Geometry: final body of the model. Coordinates: model frame, mm. A direction names the side the tool comes from. Give positions to 0.01 mm unless a question says otherwise; leave off trailing zeros. Loops run counter-clockwise (first coordinate to the right, second up) from the corner with the lowest first, then second, coordinate; pieces in that order, holes last. Notation, with made-up numbers: (73, 45) - (107, 45) arc R18 cw to (107, 73) - close; hole circle Ø11 at (74.5, 86.5). An arc over 180 degrees is marked (long way). Answer in a Markdown table with one row per item.
from build123d import *

# Parameters (mm, degrees)
F1_DEPTH = 5
F2_R     = 37.5
F3_DEPTH = 10
F4_DEPTH = 40.7
F6_DEPTH = 15


with BuildPart() as f1:
    # F0 (on Top) → F1 (new body)
    with BuildSketch(Plane.XY):
        with BuildLine():
            Line((10, -10), (41.306779, -10))
            ThreePointArc((41.306779, -10), (-39.719354, 15.120281), (37.5, -20))
            Line((37.5, -20), (0, -20))
            Line((0, -20), (0, -5))
            ThreePointArc((0, -5), (-5, 0), (0, 5))
            Line((0, 5), (0, 20))
            ThreePointArc((0, 20), (5, 25), (10, 20))
            Line((10, 20), (10, 5))
            ThreePointArc((10, 5), (15, 0), (10, -5))
            Line((10, -5), (10, -10))
        make_face()
        with BuildLine():
            ThreePointArc((37.5, -20), (39.719354, -15.120281), (41.306779, -10))
            Line((41.306779, -10), (10, -10))
            Line((10, -10), (10, -5))
            ThreePointArc((10, -5), (15, 0), (10, 5))
            Line((10, 5), (10, 20))
            ThreePointArc((10, 20), (5, 25), (0, 20))
            Line((0, 20), (0, 5))
            ThreePointArc((0, 5), (-5, 0), (0, -5))
            Line((0, -5), (0, -20))
            Line((0, -20), (37.5, -20))
        make_face()
    extrude(amount=-F1_DEPTH)

    # F2 (on face) → F3 (join)
    with BuildSketch(Plane(origin=(0, 0, -5), x_dir=(1, 0, 0), z_dir=(0, 0, -1))):
        Circle(F2_R)
    extrude(amount=F3_DEPTH)

    # F0 (on Top) → F4 (cut)
    with BuildSketch(Plane.XY):
        with BuildLine():
            ThreePointArc((37.5, -20), (39.719354, -15.120281), (41.306779, -10))
            Line((41.306779, -10), (10, -10))
            Line((10, -10), (10, -5))
            ThreePointArc((10, -5), (15, 0), (10, 5))
            Line((10, 5), (10, 20))
            ThreePointArc((10, 20), (5, 25), (0, 20))
            Line((0, 20), (0, 5))
            ThreePointArc((0, 5), (-5, 0), (0, -5))
            Line((0, -5), (0, -20))
            Line((0, -20), (37.5, -20))
        make_face()
    extrude(amount=-F4_DEPTH, mode=Mode.SUBTRACT)

    # F5 (on face) → F6 (join)
    with BuildSketch(Plane.XY):
        with BuildLine():
            ThreePointArc((-36.055513, -22.5), (-42.5, 0), (-36.055513, 22.5))
            Line((-36.055513, 22.5), (-52, 22.5))
            Line((-52, 22.5), (-52, -22.5))
            Line((-52, -22.5), (-36.055513, -22.5))
        make_face()
        with BuildLine():
            Line((-7, -22.5), (-7, 22.5))
            Line((-7, 22.5), (-36.055513, 22.5))
            ThreePointArc((-36.055513, 22.5), (-42.5, 0), (-36.055513, -22.5))
            Line((-36.055513, -22.5), (-7, -22.5))
        make_face()
    extrude(amount=F6_DEPTH)


solid = f1.part
Q1. Draft query along X for faces 5 (the flat face through (0, -12, -7)), 6 (the flat face through (0, 13, -7)), 7 (the flat face through (11, 10, 0)), 8 (the cylindrical face through (-39.046, 16.783, -2.465)). Return one class per face: pulls with the +X half, pulls with the -X half, needs draft (parallel to the pull), parting line crosses it, or undercut.
Check values:
| item | result |
|---|---|
| face 5 | undercut |
| face 6 | undercut |
| face 7 | needs draft |
| face 8 | parting line crosses it |
Q2. Cut plane B-B (z = -7.25). Output: boundary loops of the cut face in (x, y), and give its area (3 significant figures).
Check values:
| item | result |
|---|---|
| outline | (0, -20) - (0, -5) arc R5 cw to (0, 5) - (0, 20) arc R5 cw to (10, 20) - (10, 5) arc R5 cw to (10, -5) - (10, -10) - (36.14, -10) arc R37.5 ccw (long way) to (31.72, -20) - close |
| area | 3,660 mm² |
Q3. Reachability of faces 1 (the cylindrical face through (-5, 0, -7)), 2 (the flat face through (18, -20, -7)), 3 (the cylindrical face through (-34.904, 13.711, -9.93)), 4 (the flat face through (-30, -22.5, 7)) from +Z, -Z, +X, -X, +Y, -Y: full face, straight path, thin tool, end or side. Return the list, or none.
Check values:
| item | result |
|---|---|
| face 1 | +Z, -Z |
| face 2 | +Z, -Z, +X |
| face 3 | -Z |
| face 4 | +Z, +X, -X, -Y |
Q4. Cut plane C-C (x = 5). Output: boundary loops of the cut face in (y, z).
Check values:
| item | result |
|---|---|
| outline | (-42.2, -5) - (-37.17, -5) - (-37.17, -15) - (-20, -15) - (-20, 0) - (-42.2, 0) - close; (25, -15) - (37.17, -15) - (37.17, -5) - (42.2, -5) - (42.2, 0) - (25, 0) - close |
Q5. First-contact query: pin 1 (8 mm diameter, centred on y = 33.5, z = -4, fed in from -X); pin 2 (4.5 mm diameter, centred on x = 29, z = -5.5, fed in from -Y); pin 3 (1.5 mm diameter, centred on y = 15.5, z = 0, fed in from +X); pin 4 (8 mm diameter, centred on x = -4, y = -7.5, fed in from +Z). Flat tips, straight axial feed; report the tip coordinate or a pass-through.
Check values:
| item | result |
|---|---|
| pin 1 | x = -30.59 |
| pin 2 | y = -32.98 |
| pin 3 | x = 39.86 |
| pin 4 | z = 15 |
Q6. Cut plane A-A (y = 0). Output: boundary loops of the cut face in (x, z), and give its area (3 significant figures).
Check values:
| item | result |
|---|---|
| outline | (-52, 0) - (-42.5, 0) - (-42.5, -5) - (-37.5, -5) - (-37.5, -15) - (-5, -15) - (-5, 0) - (-7, 0) - (-7, 15) - (-52, 15) - close; (15, -15) - (37.5, -15) - (37.5, -5) - (42.5, -5) - (42.5, 0) - (15, 0) - close |
| area | 1,550 mm² |
Q7. Cut plane D-D (y = 35). Output: boundary loops of the cut face in (x, z).
Check values:
| item | result |
|---|---|
| outline | (-24.11, -5) - (-13.46, -5) - (-13.46, -15) - (13.46, -15) - (13.46, -5) - (24.11, -5) - (24.11, 0) - (-24.11, 0) - close |
Q8. Material intervals for line 1 along Y through (x, z) = (-37.5, 2.75); line 2 along Z through (x, y) = (25, -34); line 3 along X through (y, z) = (12.5, 7), sorted ascending.
Check values:
| item | result |
|---|---|
| line 1 | -22.5 to 22.5 |
| line 2 | -5 to 0 |
| line 3 | -52 to -7 |
